For this review, take the finished solid that the model builds, in its own axes (mm). Give positions to 0.01 mm unless a question says otherwise; leave off trailing zeros. Loops run counter-clockwise (first coordinate to the right, second up) from the corner with the lowest first, then second, coordinate; pieces in that order, holes last. Notation, with made-up numbers: (71, -18.75) - (111, -18.75) arc R10 cw to (111, -6.75) - close; hole circle Ø5 at (-19, -32.75). An arc over 180 degrees is marked (long way). Put each result on its own line as item: value. Start each with the question number.
from build123d import *

# Parameters (mm, degrees)
BOSS_EXTRUDE1_DEPTH = 1.6
SKETCH4_R           = 1.5
CUT_EXTRUDE1_DEPTH  = 54.075983269


with BuildPart() as part:
    # Sketch3 → Boss-Extrude1 (new body)
    with BuildSketch(Plane.XY):
        with BuildLine():
            Line((13.5, 36.5), (38.5, 36.5))
            Line((38.5, 36.5), (38.5, -36.5))
            Line((38.5, -36.5), (13.5, -36.5))
            Line((13.5, -36.5), (0, -36.5))
            Line((0, -36.5), (0, -13.5))
            ThreePointArc((0, -13.5), (13.5, 0), (0, 13.5))
            Line((0, 13.5), (0, 36.5))
            Line((0, 36.5), (13.5, 36.5))
        make_face()
    extrude(amount=-BOSS_EXTRUDE1_DEPTH)

    # Sketch4 → Cut-Extrude1 (cut, through all)
    with BuildSketch(Plane.XY):
        with Locations(Location((35, 33, 0), (0, 0, 180))):
            Circle(SKETCH4_R)
        with Locations((3.5, -33)):
            Circle(SKETCH4_R)
        with Locations(Location((3.5, 33, 0), (0, 0, 180))):
            Circle(SKETCH4_R)
        with Locations((28, -33)):
            Circle(SKETCH4_R)
    extrude(amount=-CUT_EXTRUDE1_DEPTH, mode=Mode.SUBTRACT)


solid = part.part
1) Mouldability with a two-part tool opening along Y and no side actions: class faces 1 (the cylindrical face through (13.497, -0.297, -0.789)), 2 (the flat face through (38.5, 1, -1)), 3 (the flat face through (20, -36.5, -1)), 4 (the cylindrical face through (2.81, 34.33, -0.79)) as released by +Y, released by -Y, zero draft, split by the parting line, or undercut.
2) Take a section at C-C on x = 35. State the section outline as (y, z) points, and give its area (3 significant figures).
3) Take a section at B-B on z = -0.7. State the section outline as (x, y) points.
4) Take a section at D-D on x = 3.5. State the section outline as (y, z) points, and give its area (3 significant figures).
5) Take a section at A-A on y = 33. State the section outline as (x, z) points, and give its area (3 significant figures).
6) Wall thickness on probe 1 along Y at (x, z) = (3.5, -0.2); probe 2 along X at (y, z) = (33, -0.5); probe 3 along Y at (x, z) = (28, -0.2): over which ranges is each line inside the solid? List them lowest first.
7) Insertion check: P1, Ø1.8, axis at x = 3.5, y = 33, coming from the +Z side. The pin has a flat end and moves straight along its axis. Give the tip position at first contact, or say it passes through.
Answers follow:
1. face 1: undercut
1. face 2: zero draft
1. face 3: released by -Y
1. face 4: undercut
2. outline: (-36.5, -1.6) - (31.5, -1.6) - (31.5, 0) - (-36.5, 0) - close; (34.5, -1.6) - (36.5, -1.6) - (36.5, 0) - (34.5, 0) - close
2. area: 112 mm2
3. outline: (0, -36.5) - (38.5, -36.5) - (38.5, 36.5) - (0, 36.5) - (0, 13.5) arc R13.5 cw to (0, -13.5) - close; hole circle Ø3 at (3.5, -33); hole circle Ø3 at (3.5, 33); hole circle Ø3 at (28, -33); hole circle Ø3 at (35, 33)
4. outline: (-36.5, -1.6) - (-34.5, -1.6) - (-34.5, 0) - (-36.5, 0) - close; (-31.5, -1.6) - (-13.04, -1.6) - (-13.04, 0) - (-31.5, 0) - close; (13.04, -1.6) - (31.5, -1.6) - (31.5, 0) - (13.04, 0) - close; (34.5, -1.6) - (36.5, -1.6) - (36.5, 0) - (34.5, 0) - close
4. area: 65.5 mm2
5. outline: (0, -1.6) - (2, -1.6) - (2, 0) - (0, 0) - close; (5, -1.6) - (33.5, -1.6) - (33.5, 0) - (5, 0) - close; (36.5, -1.6) - (38.5, -1.6) - (38.5, 0) - (36.5, 0) - close
5. area: 52.0 mm2
6. probe 1: -36.5 to -34.5, -31.5 to -13.04, 13.04 to 31.5, 34.5 to 36.5
6. probe 2: 0 to 2, 5 to 33.5, 36.5 to 38.5
6. probe 3: -36.5 to -34.5, -31.5 to 36.5
7. P1: through
